Geometry: see drawing. Coordinates: mm, zero at the bounding-box minimum. A direction names the side the tool comes from. Give positions to 0.01 mm unless a question says otherwise; leave off trailing zeros. Write each loop counter-clockwise with the first axis right and the second up, starting at its lowest first coordinate (ties: lowest second). Pieces come first, ordered by that corner, then holes. Notation, with made-up numbers: M 65.25,89 L 84.25,89 A24 ccw 84.25,122 Z; hole C 16.5,-18 d9. An arc over 180 degrees is marked long. Use a Markdown table: item, result. Add a question column.
1) Line query: line 1 (Y direction, x = 66, z = 4.4); line 2 (X direction, y = 33, z = 1.3). Output: solid intervals per line, ascending.
2) Set-up query: the marked faces 1, 2 and 3. Return all of +Z, -Z, +X, -X, +Y, -Y with unobstructed straight access to the full face (end or side cutting, diameter ignored); none if empty.
3) Pin query (flat end, axial travel): pin 1 (1.5 mm diameter, centred on x = 67, z = 3.5, fed in from -Y); pin 2 (2.5 mm diameter, centred on x = 66.5, z = 2.5, fed in from +Y). Return the tip coordinate at first contact, or that it passes through.
4) Section A-A on z = 3.8. Return the cut outline in (x, y).
5) Section B-B on y = 26.5. Return the cut outline in (x, z).
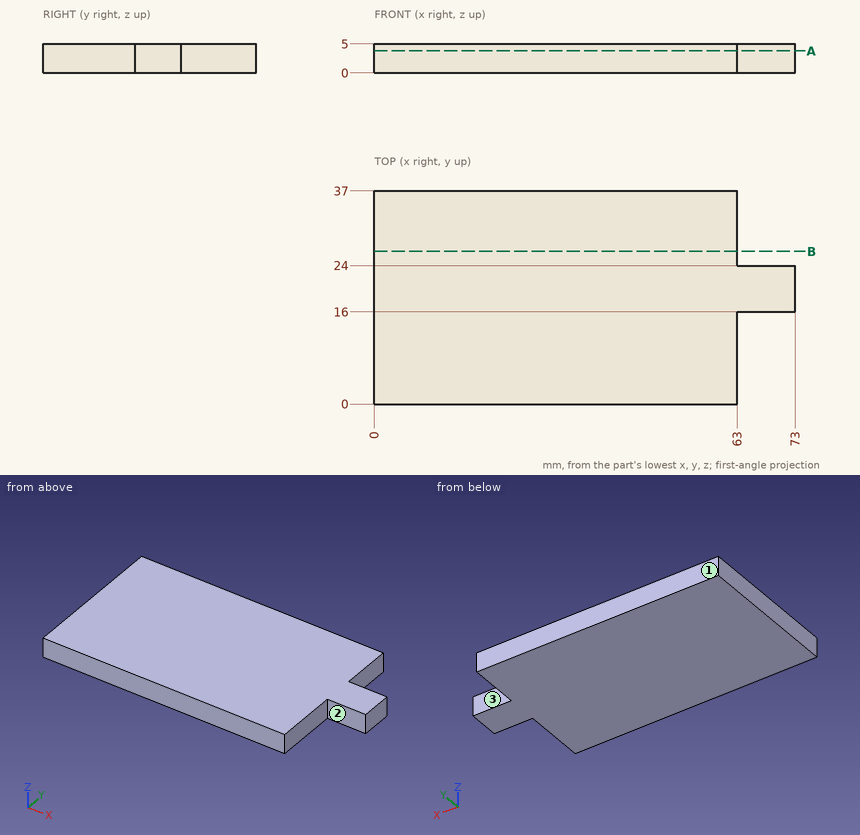
Found:
| question | item | result |
|---|---|---|
| 1 | line 1 | 16 to 24 |
| 1 | line 2 | 0 to 63 |
| 2 | face 1 | +Z, -Z, +X, -X, +Y |
| 2 | face 2 | +Z, -Z, +X, -Y |
| 2 | face 3 | +Z, -Z, +X, +Y |
| 3 | pin 1 | y = 16 |
| 3 | pin 2 | y = 24 |
| 4 | outline | M 0,0 L 63,0 L 63,16 L 73,16 L 73,24 L 63,24 L 63,37 L 0,37 Z |
| 5 | outline | M 0,0 L 63,0 L 63,5 L 0,5 Z |
